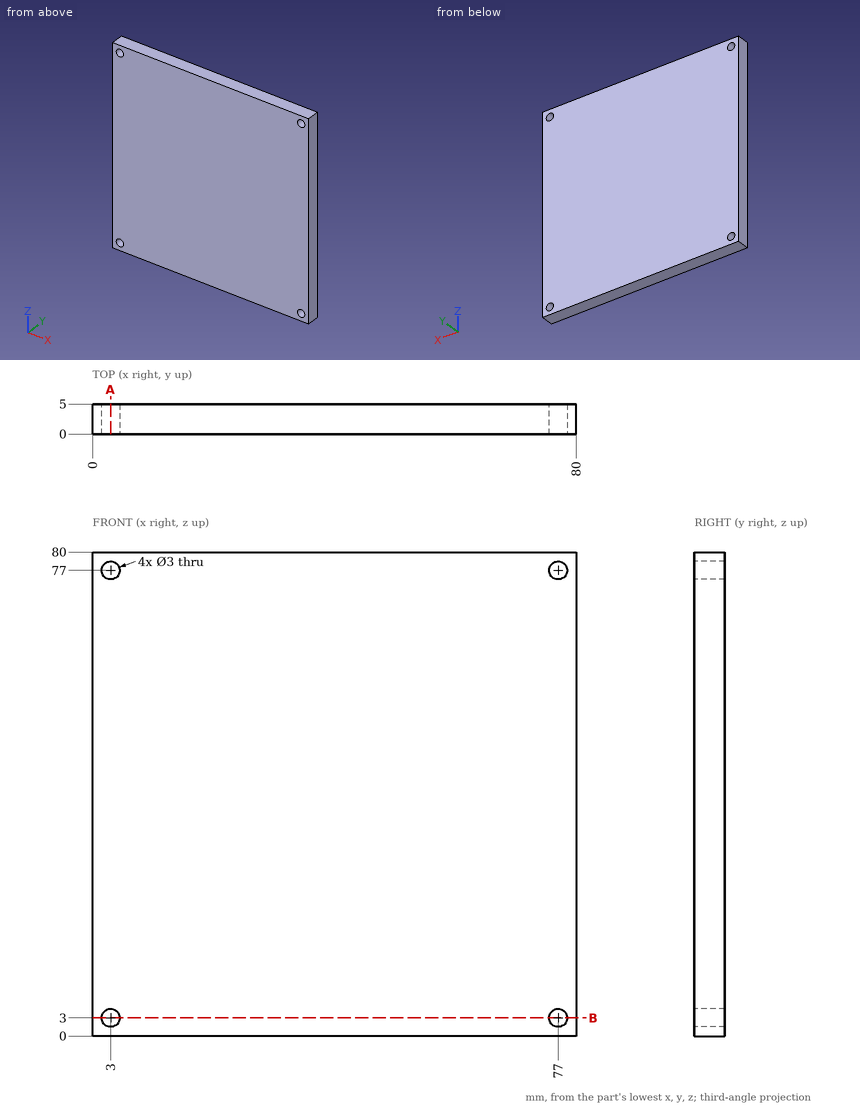
Part print with two shaded views. Sizes in mm from the minimum x, y, z corner. Coordinates: 2 decimals unless noted, no trailing zeros. Loops run counter-clockwise (first coordinate to the right, second up) from the corner with the lowest first, then second, coordinate; pieces in that order, holes last. Notation, with made-up numbers: (-8, -27) - (17, -27) arc R33 ccw to (17, 5) - close; hole circle Ø4 at (-23, 71). An arc over 180 degrees is marked (long way). Write each question's results on one line, items separated by ' | '. Start each with the question number.
Q1. Slice it at A-A on x = 3. Give the cut face in (y, z), and give its area (3 significant figures).
Q2. Drop a flat-ended pin along its axis: pin 1 Ø6 at (x, z) = (33.5, 33) entering from -Y. Give the stop position or say it passes through.
Q3. Probe line 1 along Z through (x, y) = (3, 3.4); line 2 along X through (y, z) = (4.45, 76.5). List the from-to ranges inside material, lowest first.
Q4. Slice it at B-B on z = 3. Give the cut face in (x, y), and give its area (3 significant figures).
Answer:
1) outline: (0, 0) - (5, 0) - (5, 1.5) - (0, 1.5) - close; (0, 4.5) - (5, 4.5) - (5, 75.5) - (0, 75.5) - close; (0, 78.5) - (5, 78.5) - (5, 80) - (0, 80) - close | area: 370 mm2
2) pin 1: stops at y = 0
3) line 1: z = 0 to 1.5, 4.5 to 75.5, 78.5 to 80 | line 2: x = 0 to 1.59, 4.41 to 75.59, 78.41 to 80
4) outline: (0, 0) - (1.5, 0) - (1.5, 5) - (0, 5) - close; (4.5, 0) - (75.5, 0) - (75.5, 5) - (4.5, 5) - close; (78.5, 0) - (80, 0) - (80, 5) - (78.5, 5) - close | area: 370 mm2
